```python
from build123d import *

# Parameters (mm, degrees)
BOSS_EXTRUDE1_DEPTH = 13
CUT_EXTRUDE1_DEPTH  = 10
SKETCH4_W           = 21.5
SKETCH4_H           = 26
BOSS_EXTRUDE2_DEPTH = 5
SKETCH5_R           = 3
CUT_EXTRUDE2_DEPTH  = 39


with BuildPart() as part:
    # Sketch1 → Boss-Extrude1 (new body, symmetric)
    with BuildSketch(Plane(origin=(0, 0, 0), x_dir=(1, 0, 0), z_dir=(0, 1, 0))):
        with BuildLine():
            Line((0, 0), (21.5, 0))
            Line((21.5, 0), (14.467721765, -24.012898335))
            ThreePointArc((14.467721765, -24.012898335), (13.043725458, -26.964613514), (10.741924274, -29.297444262))
            Line((10.741924274, -29.297444262), (0.20999258, -36.935988128))
            ThreePointArc((0.20999258, -36.935988128), (-8.079954607, -36.293771416), (-9.907897405, -28.182403357))
            Line((-9.907897405, -28.182403357), (0, -5.649444205))
            Line((0, -5.649444205), (0, 0))
        make_face()
    extrude(amount=BOSS_EXTRUDE1_DEPTH, both=True)

    # Sketch1_2 → Cut-Extrude1 (cut, symmetric)
    with BuildSketch(Plane(origin=(0, 0, 0), x_dir=(1, 0, 0), z_dir=(0, 1, 0))):
        with BuildLine():
            Line((0, 0), (21.5, 0))
            Line((21.5, 0), (14.467721765, -24.012898335))
            ThreePointArc((14.467721765, -24.012898335), (13.043725458, -26.964613514), (10.741924274, -29.297444262))
            Line((10.741924274, -29.297444262), (0.20999258, -36.935988128))
            ThreePointArc((0.20999258, -36.935988128), (-8.079954607, -36.293771416), (-9.907897405, -28.182403357))
            Line((-9.907897405, -28.182403357), (0, -5.649444205))
            Line((0, -5.649444205), (0, 0))
        make_face()
    extrude(amount=CUT_EXTRUDE1_DEPTH, both=True, mode=Mode.SUBTRACT)

    # Sketch4 → Boss-Extrude2 (add)
    with BuildSketch(Plane(origin=(0, 0, 0), x_dir=(-1, 0, 0), z_dir=(0, 0, -1))):
        with Locations((-10.75, 0)):
            Rectangle(SKETCH4_W, SKETCH4_H)
    extrude(amount=-BOSS_EXTRUDE2_DEPTH)

    # Sketch5 → Cut-Extrude2 (cut, through all)
    with BuildSketch(Plane(origin=(0, 0, 0), x_dir=(-1, 0, 0), z_dir=(0, 0, -1))):
        with Locations((-10.75, 0)):
            Circle(SKETCH5_R)
    extrude(amount=-CUT_EXTRUDE2_DEPTH, mode=Mode.SUBTRACT)


solid = part.part
```
Input: part model. Units: mm. Frame: model coordinates. A direction names the side the tool comes from. Coordinates: 2 decimals unless noted, no trailing zeros. Write each loop counter-clockwise with the first axis right and the second up, starting at its lowest first coordinate (ties: lowest second). Pieces come first, ordered by that corner, then holes. Notation, with made-up numbers: (43.5, -17.75) -> (88.5, -17.75) arc R23 cw to (88.5, 0.25) -> close; hole circle Ø10 at (46, 29). An arc over 180 degrees is marked (long way). Write each question's results on one line, items separated by ' | '.
Item 1: Section query C-C on x = 2. Return loops of the section in (y, z).
Conclusion:
outline: (-13, 0) -> (13, 0) -> (13, 35.64) -> (10, 35.64) -> (10, 5) -> (-10, 5) -> (-10, 35.64) -> (-13, 35.64) -> close
Item 2: Section query B-B on z = 30. Return loops of the section in (x, y).
Conclusion:
outline: (-10.43, -13) -> (9.77, -13) -> (9.77, -10) -> (-10.43, -10) -> close; (-10.43, 10) -> (9.77, 10) -> (9.77, 13) -> (-10.43, 13) -> close
Item 3: Set-up query: faces 1 (the flat face through (0, 0, 3)), 2 (the flat face through (5, -10, 21)), 3 (the flat face through (6, 13, 19)). Return all of +Z, -Z, +X, -X, +Y, -Y with unobstructed straight access to the full face (end or side cutting, diameter ignored); none if empty.
Conclusion:
face 1: -Z, -X, +Y, -Y | face 2: +Z, +X, -X | face 3: +Z, -Z, +X, -X, +Y
Item 4: Pin query (flat end, axial travel): pin 1 Ø1.5 at (x, z) = (11, 32.5) entering from -Y; pin 2 Ø6.5 at (x, y) = (9.5, -4) entering from +Z; pin 3 Ø4 at (y, z) = (-9.5, 33.5) entering from -X; pin 4 Ø3 at (y, z) = (-4, 3.5) entering from -X. Return the tip coordinate at first contact, or that it passes through.
Conclusion:
pin 1: passes through | pin 2: stops at z = 5 | pin 3: stops at x = -10.48 | pin 4: stops at x = 0
Item 5: Section query A-A on y = 0. Return loops of the section in (x, z).
Conclusion:
outline: (0, 0) -> (7.75, 0) -> (7.75, 5) -> (0, 5) -> close; (13.75, 0) -> (21.5, 0) -> (21.5, 5) -> (13.75, 5) -> close
Item 6: Material intervals for probe 1 along Y at (x, z) = (10.75, 1.6); probe 2 along Y at (x, z) = (5.5, 27.5); probe 3 along Z at (x, y) = (0.5, 0.5), sorted ascending.
Conclusion:
probe 1: y = -13 to -3, 3 to 13 | probe 2: y = -13 to -10, 10 to 13 | probe 3: z = 0 to 5
Item 7: Mould query, pull axis X, two halves, no side actions, for faces 4 (the cylindrical face through (13.131, -1.825, 2.465)), 5 (the flat face through (13, 3, 5)), 6 (the flat face through (5.5, -11.5, 33.1)). Classes: +X half, -X half, draft (parallel to the pull), parting line (faces both ways), or undercut.
Conclusion:
face 4: undercut | face 5: draft | face 6: +X half
Item 8: Section query D-D on y = -7.5. Return loops of the section in (x, z).
Conclusion:
outline: (0, 0) -> (21.5, 0) -> (21.5, 5) -> (0, 5) -> close
